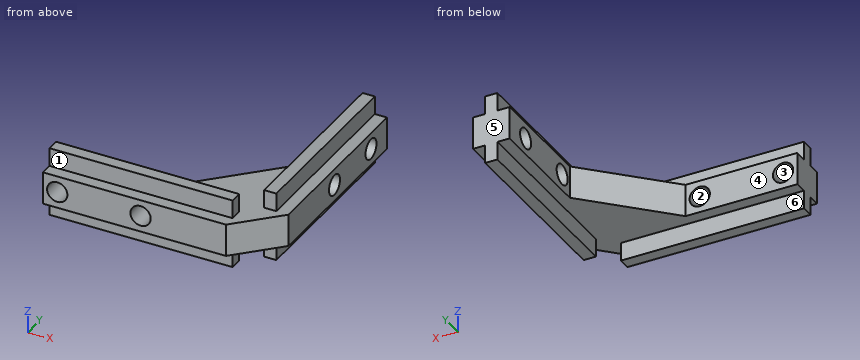
from build123d import *

# Parameters (mm, degrees)
BOSS_EXTRUDE1_DEPTH         = 4
SKETCH3_W                   = 45
SKETCH3_H                   = 3
SKETCH3_W_2                 = 3
SKETCH3_H_2                 = 45
BOSS_EXTRUDE2_DEPTH         = 4.5
BOSS_EXTRUDE3_START         = -8
SKETCH3_2_W                 = 45
SKETCH3_2_H                 = 3
SKETCH3_2_W_2               = 3
SKETCH3_2_H_2               = 45
BOSS_EXTRUDE3_DEPTH         = 4.5
TAP_DRILL_FOR_M6X1_0_TAP1_D = 5
TAP_DRILL_FOR_M6X1_0_TAP2_D = 5


with BuildPart() as part:
    # Sketch2 → Boss-Extrude1 (new, symmetric)
    with BuildSketch(Plane.XY):
        Polygon((0, 0), (45, 0), (55, 10), (55, 55), (46, 55), (46, 27.5), (27.5, 9), (0, 9), align=None)
    extrude(amount=BOSS_EXTRUDE1_DEPTH, both=True)

    # Sketch3 → Boss-Extrude2 (add)
    with BuildSketch(Plane.XY.offset(4)):
        with Locations((22.5, 4.5)):
            Rectangle(SKETCH3_W, SKETCH3_H)
        with Locations((50.5, 32.5)):
            Rectangle(SKETCH3_W_2, SKETCH3_H_2)
    extrude(amount=BOSS_EXTRUDE2_DEPTH)

    # Sketch3<2> → Boss-Extrude3 (add)
    with BuildSketch(Plane.XY.offset(4).offset(BOSS_EXTRUDE3_START)):
        with Locations((22.5, 4.5)):
            Rectangle(SKETCH3_2_W, SKETCH3_2_H)
        with Locations((50.5, 32.5)):
            Rectangle(SKETCH3_2_W_2, SKETCH3_2_H_2)
    extrude(amount=-BOSS_EXTRUDE3_DEPTH)

    # Tap Drill for M6x1.0 Tap1 (through all)
    with Locations(Plane.ZY.offset(-46)):
        with Locations((0, 31), (0, 47.69)):
            Hole(TAP_DRILL_FOR_M6X1_0_TAP1_D / 2)

    # Tap Drill for M6x1.0 Tap2 (through all)
    with Locations(Plane(origin=(0, 9, 0), x_dir=(1, 0, 0), z_dir=(0, 1, 0))):
        with Locations((24, 0), (3.5, 0)):
            Hole(TAP_DRILL_FOR_M6X1_0_TAP2_D / 2)


solid = part.part
Geometry check sheet. Reference: the model listing, model coordinates, mm. Face numbers are marked on the shaded views. A direction names the side the tool comes from. Round coordinates to 2 decimals unless told otherwise and drop trailing zeros. Order: outer loops, then holes, each group sorted by start corner. A loop starts at its lowest first (then second) coordinate and runs counter-clockwise, first axis right, second up. Notation, with made-up numbers: M 29,83 L 47,83 A12 cw 47,106 Z; hole C 30.25,-3.75 d10. An arc over 180 degrees is marked long. Write each question's results on one line, items separated by ' | '. Start each with the question number.
1. Draft check along Z on the marked faces 1, 2 and 3. Enter one of: pulls with the +Z half, pulls with the -Z half, needs draft (parallel to the pull), parting line crosses it, or undercut.
2. Cross-section at A-A on z = 0. Record the boundary of the cut face in (x, y), plus the area to 3 significant figures.
3. Cross-section at C-C on y = 5. Record the boundary of the cut face in (x, z).
4. Material ranges on L1, parallel to Y at x = 50.25, z = 0; L2, parallel to Y at x = 24.5, z = -3.5; L3, parallel to X at y = 44, z = -0.75, recorded low to high. Write a range as from..to.
5. Cross-section at D-D on x = 24. Record the boundary of the cut face in (y, z).
6. Cross-section at B-B on y = 31. Record the boundary of the cut face in (x, z).
7. Go/stop test with flat-tipped pins: P1, Ø3.5, axis at x = 24.5, z = -6, coming from the +Y side; P2, Ø2, axis at y = 43.5, z = -7, coming from the +X side; P3, Ø4, axis at x = 42, z = -2.5, coming from the +Y side; P4, Ø5, axis at x = 28, z = -4, coming from the -Y side. Record where each tip stops, or that it passes through.
8. Set-up check for the marked faces 4, 5 and 6: record each of +Z, -Z, +X, -X, +Y, -Y from which the full face is reachable in a straight line by a thin tool's end or side.
Resolved:
1) face 1: needs draft | face 2: undercut | face 3: undercut
2) outline: M 0,0 L 1,0 L 1,9 L 0,9 Z; M 6,0 L 21.5,0 L 21.5,9 L 6,9 Z; M 26.5,0 L 45,0 L 55,10 L 55,28.5 L 46,28.5 L 46,27.5 L 27.5,9 L 26.5,9 Z; M 46,33.5 L 55,33.5 L 55,45.19 L 46,45.19 Z; M 46,50.19 L 55,50.19 L 55,55 L 46,55 Z | area: 850 mm2
3) outline: M 0,-8.5 L 45,-8.5 L 45,-4 L 50,-4 L 50,4 L 45,4 L 45,8.5 L 0,8.5 Z; hole C 3.5,0 d5; hole C 24,0 d5
4) L1: 5.25..28.5, 33.5..45.19, 50.19..55 | L2: 0..9 | L3: 46..55
5) outline: M 0,-4 L 3,-4 L 3,-8.5 L 6,-8.5 L 6,-4 L 9,-4 L 9,-2.5 L 0,-2.5 Z; M 0,2.5 L 9,2.5 L 9,4 L 6,4 L 6,8.5 L 3,8.5 L 3,4 L 0,4 Z
6) outline: M 46,-4 L 49,-4 L 49,-8.5 L 52,-8.5 L 52,-4 L 55,-4 L 55,-2.5 L 46,-2.5 Z; M 46,2.5 L 55,2.5 L 55,4 L 52,4 L 52,8.5 L 49,8.5 L 49,4 L 46,4 Z
7) P1: y = 6 | P2: x = 52 | P3: y = 25.5 | P4: y = 0
8) face 4: +Z, -Z, -X, +Y | face 5: +Z, -Z, +X, -X, +Y | face 6: -Z, +X, -X, +Y
